Read the model definition and answer for the solid it produces. Units are mm, in the model's axes. Face numbers are marked on the shaded views. A direction names the side the tool comes from. Round coordinates to 2 decimals unless told otherwise and drop trailing zeros. Write each loop counter-clockwise with the first axis right and the second up, starting at its lowest first coordinate (ties: lowest second). Pieces come first, ordered by that corner, then holes.
from build123d import *

# Parameters (mm, degrees)
F0_W     = 508
F0_H     = 302.9659508712
F1_DEPTH = 50.8
F2_W     = 77.5359706879
F2_H     = 302.9659508712
F3_DEPTH = 175.26
F4_W     = 71.7851296759
F4_H     = 39.8045896537
F4_W_2   = 50.8
F4_H_2   = 39.8045703769
F4_W_3   = 55.2871824002
F4_H_3   = 38.1124727428
F4_W_4   = 66.2858231544
F4_H_4   = 40.2276038176
F5_DEPTH = 508


with BuildPart() as f1:
    # F0 (on Front) → F1 (new body)
    with BuildSketch(Plane.XZ):
        with Locations((-254, 151.4829754356)):
            Rectangle(F0_W, F0_H)
    extrude(amount=F1_DEPTH)

    # F2 (on face) → F3 (join)
    with BuildSketch(Plane(origin=(0, 0, 0), x_dir=(-1, 0, 0), z_dir=(0, 1, 0))):
        with Locations((469.2320146561, 151.4829754356)):
            Rectangle(F2_W, F2_H)
    extrude(amount=F3_DEPTH)

    # F4 (on face) → F5 (join)
    with BuildSketch(Plane(origin=(-508, 0, 0), x_dir=(0, -1, 0), z_dir=(-1, 0, 0))):
        with Locations((-139.3674351621, 283.0636560443)):
            Rectangle(F4_W, F4_H)
        with Locations((25.4, 19.9022851884)):
            Rectangle(F4_W_2, F4_H_2)
        with Locations((-147.6164087999, 19.0562363714)):
            Rectangle(F4_W_3, F4_H_3)
        with Locations((17.6570884228, 282.8521489623)):
            Rectangle(F4_W_4, F4_H_4)
    extrude(amount=F5_DEPTH)


solid = f1.part
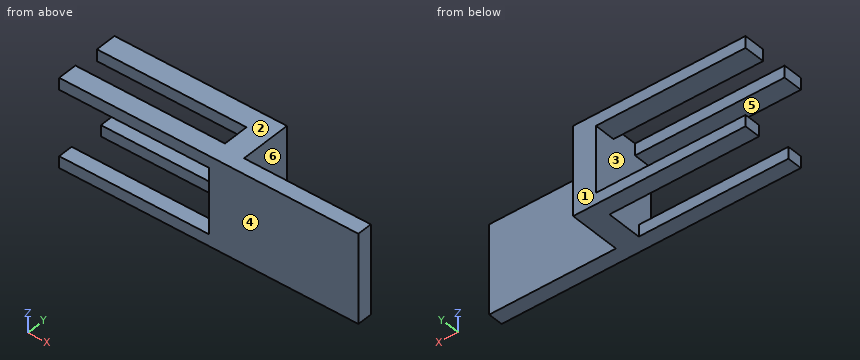
Q1. Which of the six approach directions +Z, -Z, +X, -X, +Y, -Y give full straight-line access (tool end or side, diameter ignored) to the marked faces 4, 5 and 6?
Verdict:
face 4: +Z, -Z, +X, -X, -Y
face 5: -X, +Y, -Y
face 6: +Z, -Z, +X, +Y
Q2. Section D-D (x = -202) is taken. Determine the outline of the cut face in (y, z).
Verdict:
outline: (-50.8, 0) - (0, 0) - (0, 302.97) - (-50.8, 302.97) - close
Q3. Straight lines are drawn through the part: probe 1 along Z at (x, y) = (-775, -13); probe 2 along Z at (x, y) = (-531, 144); probe 3 along X at (y, z) = (-28, 237.5). For each, find the intervals that lie inside material, in ascending order.
Verdict:
probe 1: z = 0 to 39.8, 262.74 to 302.97
probe 2: z = 0 to 38.11, 263.16 to 302.97
probe 3: x = -508 to 0
Q4. Determine the mould class of the marked faces 1, 2 and 3 for opening direction Z: pulls with the +Z half, pulls with the -Z half, needs draft (parallel to the pull), parting line crosses it, or undercut.
Verdict:
face 1: needs draft
face 2: pulls with the +Z half
face 3: undercut
Q5. Section B-B (y = -26) is taken. Determine the outline of the cut face in (x, z), then the cut area to 3 significant figures.
Verdict:
outline: (-1016, 0) - (0, 0) - (0, 302.97) - (-1016, 302.97) - (-1016, 262.74) - (-508, 262.74) - (-508, 39.8) - (-1016, 39.8) - close
area: 195,000 mm2
Q6. Flat-ended cylindrical pins translate along their axes: pin 1 Ø12 at (y, z) = (14, 262) entering from +X; pin 2 Ø1 at (y, z) = (118, 227.5) entering from -X; pin 3 Ø21.5 at (x, y) = (-693, 136.5) entering from -Z. Find the tip coordinate at first contact, or state that the pin passes through.
Verdict:
pin 1: stops at x = -430.46
pin 2: stops at x = -508
pin 3: stops at z = 0
Q7. Section A-A (x = -691) is taken. Determine the outline of the cut face in (y, z), then the cut area to 3 significant figures.
Verdict:
outline: (-50.8, 0) - (0, 0) - (0, 39.8) - (-50.8, 39.8) - close; (-50.8, 262.74) - (15.49, 262.74) - (15.49, 302.97) - (-50.8, 302.97) - close; (103.47, 263.16) - (175.26, 263.16) - (175.26, 302.97) - (103.47, 302.97) - close; (119.97, 0) - (175.26, 0) - (175.26, 38.11) - (119.97, 38.11) - close
area: 9,650 mm2
Q8. Section C-C (z = 116) is taken. Determine the outline of the cut face in (x, y), then the cut area to 3 significant figures.
Verdict:
outline: (-508, -50.8) - (0, -50.8) - (0, 0) - (-430.46, 0) - (-430.46, 175.26) - (-508, 175.26) - close
area: 39,400 mm2
